Autodesk Fusion 360 part; units mm, degrees
sketch "Sketch1" plane through (0, 0, 0) normal (0, 1, 0) x (1, 0, 0)
  line L0 (-120, 0) -> (-20, 0)
  line L1 (10, 17.3205) -> (60, 103.923)
  arc A0 (60, 103.923) -> (-120, 0) centre (0, 0) ccw
  arc A1 (10, 17.3205) -> (-20, 0) centre (0, 0) ccw
  dimension "d57" = 240
  dimension "d58" = 120
  dimension "d59" = 40
extrude "Extrude3" add sketch "Sketch1" along normal blind 10
sketch "Sketch9" plane through (0, 0, 0) normal (0, 0, 1) x (1, 0, 0)
  line L0 (-120, 0) -> (-20, 0)
  line L1 (-20, 0) -> (-20, 10)
  line L2 (-20, 10) -> (-120, 10)
  line L3 (-120, 10) -> (-120, 0)
  line L4 (-120, 10) -> (-10, 10)
  line L5 (-10, 10) -> (-10, 6)
  line L6 (-10, 6) -> (-120, 6)
  line L7 (-120, 6) -> (-120, 10)
  dimension "d60" = 4
extrude "Extrude8" add sketch "Sketch9" along normal blind 10 contours L1 L2 L3 L4 L6 L7
sketch "Sketch12" plane through (0, 0, 0) normal (0.866, 0, 0.5) x (0.5, 0, -0.866)
  line L0 (20, 0) -> (120, 0)
  line L1 (120, 0) -> (120, 10)
  line L2 (120, 10) -> (20, 10)
  line L3 (20, 10) -> (20, 0)
  line L4 (20, 0) -> (130, 0)
  line L5 (130, 0) -> (130, 6)
  line L6 (130, 6) -> (20, 6)
  line L7 (20, 6) -> (20, 0)
  dimension "d63" = 6
extrude "Extrude9" add sketch "Sketch12" along normal blind 10 contours L0 L1 L3 L4 L6 L7
sketch "Sketch13" plane through (0, 10, 0) normal (0, 1, 0) x (-1, 0, 0)
  arc A0 (-60, -103.923) -> (120, 0) centre (0, 0) ccw
  arc A1 (-10, -17.3205) -> (20, 0) centre (0, 0) ccw
  line L0 (-10, -17.3205) -> (-60, -103.923)
  line L1 (120, 0) -> (120, 10)
  line L2 (120, 10) -> (20, 10)
  line L3 (20, 10) -> (20, 0)
  point P0 (85, 5)
  point P1 (55, 5)
  dimension "d178" = 30
  dimension "d179" = 35
hole "Hole1" at (-85, 10, 5) at (-55, 10, 5) direction (0, -1, 0) diameter 4 depth 4 tip angle 118 countersink diameter 6 countersink angle 90
sketch "Sketch14" plane through (0, 6, 0) normal (0, 1, 0) x (-1, 0, 0)
  line L0 (-60, -103.923) -> (-10, -17.3205)
  line L1 (-10, -17.3205) -> (-18.6603, -12.3205)
  line L2 (-18.6603, -12.3205) -> (-68.6603, -98.923)
  line L3 (-68.6603, -98.923) -> (-60, -103.923)
  line L4 (-14.3301, -14.8205) -> (-64.3301, -101.423) construction
  point P0 (-31.8301, -45.1314)
  point P1 (-46.8301, -71.1122)
  dimension "d75" = 35
  dimension "d76" = 35
hole "Hole2" at (31.8301, 6, -45.1314) at (46.8301, 6, -71.1122) direction (0, -1, 0) diameter 4 depth 15 tip angle 118
sketch "Sketch15" plane through (0, 10, 0) normal (0, 1, 0) x (-1, 0, 0)
  arc A0 (-60, -103.923) -> (120, 0) centre (0, 0) ccw
  arc A1 (-10, -17.3205) -> (20, 0) centre (0, 0) ccw
  line L0 (-10, -17.3205) -> (-60, -103.923)
  line L1 (0, 0) -> (60, -103.923) construction
  line L2 (20, 0) -> (120, 0)
  line L3 (56.6506, -48.1218) -> (13.3494, -73.1218) construction
  line L4 (57.1962, -87.0666) -> (46.8038, -93.0666) construction
  circle A2 centre (85, 5) radius 3
  circle A3 centre (55, 5) radius 3
  line L5 (120, 0) -> (120, 10)
  line L6 (120, 10) -> (20, 10)
  line L7 (20, 10) -> (20, 0)
  dimension "d80" = 60
  dimension "d81" = 50
  dimension "d82" = 25
  dimension "d83" = 50
  dimension "d95" = 6
  dimension "d96" = 12
  dimension "d97" = 34
sketch "Sketch16" plane through (0, 10, 0) normal (0, 1, 0) x (-1, 0, 0)
  line L0 (120, 0) -> (120, 10)
  line L1 (20, 0) -> (20, 10)
  line L2 (-10, -17.3205) -> (-18.6603, -12.3205)
  line L3 (-60, -103.923) -> (-68.6603, -98.923)
  line L4 (120, 5) -> (20, 5) construction
  line L5 (-14.3301, -14.8205) -> (-64.3301, -101.423) construction
  line L6 (-11.0289, -109.1025) -> (-97.6314, -59.1025) construction
  line L7 (100, -45) -> (100, 55) construction
  dimension "d98" = 100
  dimension "d99" = 50
  dimension "d100" = 20
  dimension "d101" = 20
  dimension "d102" = 100
  dimension "d103" = 50
sketch "Sketch17" plane through (0, 0, 0) normal (0, -1, 0) x (1, 0, 0)
  circle A0 centre (31.8301, -45.1314) radius 2
  circle A1 centre (46.8301, -71.1122) radius 2
  arc A2 (-120, 0) -> (60, -103.923) centre (0, 0) ccw
  line L0 (60, -103.923) -> (68.6603, -98.923)
  line L1 (68.6603, -98.923) -> (18.6603, -12.3205)
  line L2 (18.6603, -12.3205) -> (10, -17.3205)
  arc A3 (-20, 0) -> (10, -17.3205) centre (0, 0) ccw
  line L3 (-20, 0) -> (-120, 0)
sketch "Sketch18" plane through (0, 0, 0) normal (0, -1, 0) x (1, 0, 0)
  point P0 (-100, -45)
  point P1 (11.0289, -109.1025)
  point P2 (-100, -45)
  point P3 (11.0289, -109.1025)
sketch "Sketch23" plane through (0, 10, 0) normal (0, 1, 0) x (-1, 0, 0)
  arc A0 (-60, -103.923) -> (120, 0) centre (0, 0) ccw
  arc A1 (-10, -17.3205) -> (20, 0) centre (0, 0) ccw
  line L0 (0, 0) -> (60, -103.923) construction
  line L1 (91.8013, -59.0045) -> (5.1987, -109.0045) construction
  line L2 (15.6891, -97.1743) -> (76.3109, -62.1743)
  arc A2 (76.3109, -62.1743) -> (71.3109, -53.5141) centre (73.8109, -57.8442) ccw
  line L3 (71.3109, -53.5141) -> (10.6891, -88.5141)
  arc A3 (10.6891, -88.5141) -> (15.6891, -97.1743) centre (13.1891, -92.8442) ccw
  line L4 (13.1891, -92.8442) -> (73.8109, -57.8442) construction
  circle A4 centre (85, 5) radius 3
  circle A5 centre (55, 5) radius 3
  line L5 (120, 0) -> (120, 10)
  line L6 (120, 10) -> (20, 10)
  line L7 (20, 10) -> (20, 0)
  dimension "d147" = 35
  dimension "d148" = 70
  dimension "d149" = 5
  dimension "d150" = 82
  dimension "d184" = 100
  dimension "d185" = 50
  dimension "d186" = 97
  dimension "d187" = 109.1284
hole "Hole5" at (-91.8013, 10, -59.0045) at (-5.1987, 10, -109.0045) direction (0, -1, 0) diameter 4.5 depth 42.794 tip angle 180 countersink diameter 6 countersink angle 90
extrude "Extrude15" cut sketch "Sketch23" against normal blind 150 contours L2 A2 L3 A3
sketch "Sketch24" plane through (0, 0, 0) normal (0, -1, 0) x (1, 0, 0)
  line L0 (-15.6891, -97.1743) -> (-76.3109, -62.1743)
  arc A0 (-71.3109, -53.5141) -> (-76.3109, -62.1743) centre (-73.8109, -57.8442) ccw
  line L1 (-71.3109, -53.5141) -> (-10.6891, -88.5141)
  arc A1 (-15.6891, -97.1743) -> (-10.6891, -88.5141) centre (-13.1891, -92.8442) ccw
  circle A2 centre (-91.8013, -59.0045) radius 2.25
  circle A3 centre (-5.1987, -109.0045) radius 2.25
  circle A4 centre (31.8301, -45.1314) radius 2
  circle A5 centre (46.8301, -71.1122) radius 2
  arc A6 (-120, 0) -> (60, -103.923) centre (0, 0) ccw
  line L2 (60, -103.923) -> (68.6603, -98.923)
  line L3 (68.6603, -98.923) -> (18.6603, -12.3205)
  line L4 (18.6603, -12.3205) -> (10, -17.3205)
  arc A7 (-20, 0) -> (10, -17.3205) centre (0, 0) ccw
  line L5 (-20, 0) -> (-120, 0)
  line L6 (10, -17.3205) -> (60, -103.923) construction
  line L7 (0, 0) -> (-70, 0) construction
  line L8 (0, 0) -> (35, -60.6218) construction
  line L9 (35, -60.6218) -> (17.6795, -70.6218) construction
  line L10 (-70, 0) -> (-70, -20) construction
  dimension "d153" = 70
  dimension "d154" = 70
  dimension "d155" = 20
  dimension "d161" = 20
hole "Hole6" at (17.6795, 0, -70.6218) at (-70, 0, -20) direction (0, 1, 0) diameter 4 depth 42.794 tip angle 180 countersink diameter 6 countersink angle 90
sketch "Sketch25" plane through (0, 10, 0) normal (0, 1, 0) x (-1, 0, 0)
  circle A0 centre (-17.6795, -70.6218) radius 2
  circle A1 centre (70, -20) radius 2
  line L0 (76.3109, -62.1743) -> (15.6891, -97.1743)
  arc A2 (10.6891, -88.5141) -> (15.6891, -97.1743) centre (13.1891, -92.8442) ccw
  line L1 (10.6891, -88.5141) -> (71.3109, -53.5141)
  arc A3 (76.3109, -62.1743) -> (71.3109, -53.5141) centre (73.8109, -57.8442) ccw
  circle A4 centre (91.8013, -59.0045) radius 3
  circle A5 centre (5.1987, -109.0045) radius 3
  circle A6 centre (85, 5) radius 3
  circle A7 centre (55, 5) radius 3
  arc A8 (-60, -103.923) -> (120, 0) centre (0, 0) ccw
  line L2 (120, 0) -> (120, 10)
  line L3 (120, 10) -> (20, 10)
  line L4 (20, 10) -> (20, 0)
  arc A9 (-10, -17.3205) -> (20, 0) centre (0, 0) ccw
  line L5 (-10, -17.3205) -> (-60, -103.923)
  line L6 (54.3205, -54.0859) -> (19.6795, -74.0859) construction
  line L7 (19.6795, -74.0859) -> (-0.3205, -39.4449) construction
  line L8 (-0.3205, -39.4449) -> (34.3205, -19.4449) construction
  line L9 (34.3205, -19.4449) -> (54.3205, -54.0859) construction
  line L10 (0, 0) -> (60, -103.923)
  line L11 (71.3109, -53.5141) -> (10.6891, -88.5141)
  line L12 (47.4904, -52.2558) -> (21.5096, -67.2558)
  line L13 (21.5096, -67.2558) -> (6.5096, -41.275)
  line L14 (6.5096, -41.275) -> (32.4904, -26.275)
  line L15 (32.4904, -26.275) -> (47.4904, -52.2558)
  point P0 (54.3205, -54.0859)
  point P1 (34.3205, -19.4449)
  point P2 (-0.3205, -39.4449)
  point P3 (19.6795, -74.0859)
  dimension "d162" = 40
  dimension "d163" = 40
  dimension "d164" = 20
  dimension "d165" = 8
  dimension "d169" = 5
  dimension "d170" = 5
  dimension "d172" = 5
  dimension "d173" = 5
hole "Hole7" at (-54.3205, 10, -54.0859) at (-34.3205, 10, -19.4449) at (0.3205, 10, -39.4449) at (-19.6795, 10, -74.0859) direction (0, -1, 0) diameter 4 depth 20 tip angle 118
extrude "Extrude16" cut sketch "Sketch25" against normal blind 40 contours L10 L12 L13 L14 | L10 L12 L14 L15
equation "d82 = d81 / 2"
equation "d96 = d95 * 2"
equation "d99 = d98 / 2"
equation "d101 = d100"
equation "d102 = d98"
equation "d103 = d99"
equation "d148 = d147 * 2"
equation "d164 = d163 / 2"
equation "d185 = d184 / 2"
Work out the finished part from the listing and answer in its coordinate system (mm). A direction names the side the tool comes from. Give positions to 0.01 mm unless a question says otherwise; leave off trailing zeros. Loops run counter-clockwise (first coordinate to the right, second up) from the corner with the lowest first, then second, coordinate; pieces in that order, holes last. Notation, with made-up numbers: (12.25, 70.25) - (19.25, 70.25) arc R9 ccw to (19.25, 78.25) - close; hole circle Ø1 at (-25, 5.25). An arc over 180 degrees is marked (long way). Answer in a Markdown table with one row per item. Add a question column.
Q1. The part is cut by section C-C (z = -78). Determine the outline of the cut face in (x, y), and give its area (3 significant figures).
Q2. The part is cut by section B-B (x = -85). Determine the outline of the cut face in (y, z).
Q3. The part is cut by section D-D (z = -15). Determine the outline of the cut face in (x, y).
Q4. The part is cut by section A-A (z = 5). Determine the outline of the cut face in (x, y), and give its area (3 significant figures).
Q5. A tool of negligible diameter and unlimited length cuts with its end or side. For faces 1 (the flat face through (-31, 10, -70)), 2 (the flat face through (40, 6, -59)), 3 (the flat face through (-19.32, 5.07, -33.88)), 4 (the flat face through (-71, 8, 10)), 5 (the flat face through (-71, 3, 0)), from which of +Z, -Z, +X, -X, +Y, -Y can it reach the whole face along a straight path? Write none if from no direction.
Q6. Consider line 1 along X through (y, z) = (7.1, 5); line 2 along Z through (x, y) = (-25, 2); line 3 along X through (y, z) = (4, -39.5). Determine where each line is inside the solid, lowest interval first.
Q7. Determine the mould class of faces 6 (the flat face through (-120, 8, 5)), 7 (the flat face through (-69, 6, 5)), 8 (the cylindrical face through (-72, 6, -20)), 9 (the flat face through (43.3, 3, -55)) for opening direction X: released by +X, released by -X, zero draft, split by the parting line, or undercut.
Q8. Each of these flat-tipped pins is pushed along its axis until it touches: P1, Ø1.5, axis at y = 8.5, z = -86.5, coming from the +X side; P2, Ø1.8, axis at x = -60, y = 2, coming from the +Z side; P3, Ø3, axis at x = -19.68, z = -74.09, coming from the -Y side; P4, Ø1.2, axis at y = 7.5, z = 4.5, coming from the +X side. Where does it stop, or does it pass through?
Solution:
| question | item | result |
|---|---|---|
| 1 | outline | (-91.19, 0) - (-48.9, 0) - (-48.9, 10) - (-91.19, 10) - close; (-28.9, 0) - (56.58, 0) - (56.58, 6) - (45.03, 6) - (45.03, 10) - (-28.9, 10) - close |
| 1 | area | 1,230 mm² |
| 2 | outline | (0, -84.71) - (10, -84.71) - (10, 2) - (9, 3) - (6, 3) - (6, 0) - (0, 0) - close; (6, 7) - (9, 7) - (10, 8) - (10, 10) - (6, 10) - close |
| 3 | outline | (-119.06, 0) - (-13.23, 0) - (-13.23, 10) - (-119.06, 10) - close; (14.02, 0) - (20.21, 0) - (20.21, 6) - (14.02, 6) - close |
| 4 | outline | (-120, 6) - (-87, 6) - (-87, 9) - (-88, 10) - (-120, 10) - close; (-83, 6) - (-57, 6) - (-57, 9) - (-58, 10) - (-82, 10) - (-83, 9) - close; (-53, 6) - (-20, 6) - (-20, 10) - (-52, 10) - (-53, 9) - close |
| 4 | area | 366 mm² |
| 5 | face 1 | +Z, -Z, +X, -X, +Y |
| 5 | face 2 | +Z, +X, +Y |
| 5 | face 3 | +Y, -Y |
| 5 | face 4 | +Z, +X, -X, +Y, -Y |
| 5 | face 5 | +Z, +X, -X, -Y |
| 6 | line 1 | x = -120 to -87, -83 to -57, -53 to -20 |
| 6 | line 2 | z = -117.37 to -91.8, -80.25 to -65.24, -30.6 to 0 |
| 6 | line 3 | x = -113.31 to -40.13, -9.58 to -1.68, 2.32 to 34.35 |
| 7 | face 6 | released by -X |
| 7 | face 7 | zero draft |
| 7 | face 8 | undercut |
| 7 | face 9 | released by +X |
| 8 | P1 | stops at x = 50.37 |
| 8 | P2 | stops at z = 0 |
| 8 | P3 | passes through |
| 8 | P4 | stops at x = -20 |
